from build123d import *

# Parameters (mm, degrees)
F0_R     = 150
F0_R_2   = 11.25
F0_R_3   = 8.25
F0_R_4   = 24.5
F1_DEPTH = 24


with BuildPart() as f1:
    # F0 (on Top) → F1 (new body)
    with BuildSketch(Plane.XY):
        Circle(F0_R)
        with Locations((-42.426407, -42.426407)):
            Circle(F0_R_2, mode=Mode.SUBTRACT)
        with Locations((0, -135)):
            Circle(F0_R_3, mode=Mode.SUBTRACT)
        with Locations((42.426407, -42.426407)):
            Circle(F0_R_2, mode=Mode.SUBTRACT)
        with Locations((-135, 0)):
            Circle(F0_R_3, mode=Mode.SUBTRACT)
        with Locations((-42.426407, 42.426407)):
            Circle(F0_R_2, mode=Mode.SUBTRACT)
        Circle(F0_R_4, mode=Mode.SUBTRACT)
        with Locations((42.426407, 42.426407)):
            Circle(F0_R_2, mode=Mode.SUBTRACT)
        with Locations((135, 0)):
            Circle(F0_R_3, mode=Mode.SUBTRACT)
        with Locations((0, 135)):
            Circle(F0_R_3, mode=Mode.SUBTRACT)
    extrude(amount=-F1_DEPTH)


solid = f1.part
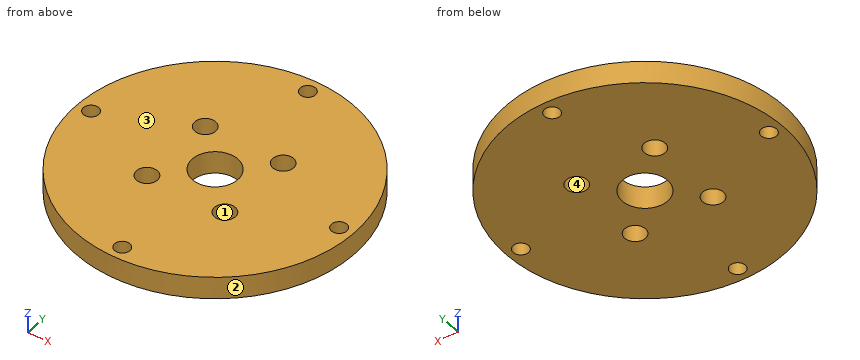
Verification items for the finished model (mm, model axes). Face numbers are marked on the shaded views. Give positions to 0.01 mm unless a question says otherwise; leave off trailing zeros. Order: outer loops, then holes, each group sorted by start corner. A loop starts at its lowest first (then second) coordinate and runs counter-clockwise, first axis right, second up. Notation, with made-up numbers: M 12,29 L 40,29 A19 ccw 40,35 Z; hole C 1.5,18.25 d7. An arc over 180 degrees is marked long. Answer as a JSON object with one key per item and string values. Group by question number.
1) Depth check by flat-ended pin: pin 1 Ø1.5 at (y, z) = (-56, -12) entering from +X; pin 2 Ø15 at (x, y) = (135, 0) entering from +Z; pin 3 Ø5 at (y, z) = (22.5, -11.5) entering from -X; pin 4 Ø2 at (x, z) = (101.5, -8) entering from -Y. Enter the tip coordinate at first touch or a pass-through.
2) Scan lines: line 1 along Y through (x, z) = (0, -5.5); line 2 along X through (y, z) = (-43, -4); line 3 along Y through (x, z) = (52.5, -11.5). Record each from-to range of solid material in increasing order. Write a range as [from, to].
3) Mould release check, pull along X, two halves, no side actions. Record for the marked faces 1, 2, 3 and 4: released by +X, released by -X, zero draft, split by the parting line, or undercut.
4) Cross-section at A-A (x = 0). Enter the section's corners in (y, z).
5) Cross-section at C-C (y = -46). Enter the section's corners in (x, z).
6) Cross-section at D-D (z = -10). Give the number of separate pieces and of enclosed holes in the cut face, then the cut area to 3 significant figures.
Result sheet:
{
 "1": {"pin 1": "stops at x = 139.45", "pin 2": "passes through", "pin 3": "stops at x = -148.66", "pin 4": "stops at y = -111.35"},
 "2": {"line 1": "y = [-150, -143.25], [-126.75, -24.5], [24.5, 126.75], [143.25, 150]", "line 2": "x = [-143.7, -53.66], [-31.19, 31.19], [53.66, 143.7]", "line 3": "y = [-140.51, -47.43], [-37.42, 37.42], [47.43, 140.51]"},
 "3": {"face 1": "undercut", "face 2": "split by the parting line", "face 3": "zero draft", "face 4": "undercut"},
 "4": {"outline": "M -150,-24 L -143.25,-24 L -143.25,0 L -150,0 Z; M -126.75,-24 L -24.5,-24 L -24.5,0 L -126.75,0 Z; M 24.5,-24 L 126.75,-24 L 126.75,0 L 24.5,0 Z; M 143.25,-24 L 150,-24 L 150,0 L 143.25,0 Z"},
 "5": {"outline": "M -142.77,-24 L -53.09,-24 L -53.09,0 L -142.77,0 Z; M -31.76,-24 L 31.76,-24 L 31.76,0 L -31.76,0 Z; M 53.09,-24 L 142.77,-24 L 142.77,0 L 53.09,0 Z"},
 "6": {"separate pieces": "1", "enclosed holes": "9", "area": "66,400 mm2"}
}
